Verification items for the finished model (mm, model axes). A direction names the side the tool comes from. Give positions to 0.01 mm unless a question says otherwise; leave off trailing zeros. Loops run counter-clockwise (first coordinate to the right, second up) from the corner with the lowest first, then second, coordinate; pieces in that order, holes last. Notation, with made-up numbers: M 16,-10.5 L 57,-10.5 A24 ccw 57,26.5 Z; hole C 39.25,-13 d6. An arc over 180 degrees is marked long. Use CSV: the item, a comma, the result in double quotes.
from build123d import *

# Parameters (mm, degrees)
SKETCH1_W         = 67.6
SKETCH1_H         = 30
SUBSTRATE_DEPTH   = 1.4
SKETCH2_R         = 1
SKETCH2_R_2       = 0.75
SKETCH2_R_3       = 1.75
CUTOUTS_DEPTH     = 2
SKETCH3_W         = 12.009016129
SKETCH3_H         = 11.886366808
SKETCH3_W_2       = 10.970861006
SKETCH3_H_2       = 9.979144757
CHIPS_DEPTH       = 0.3
SKETCH4_W         = 3.027468224
SKETCH4_H         = 1.391658781
SKETCH4_H_2       = 1.39165878
SKETCH4_W_2       = 1.760997679
SKETCH4_H_3       = 0.651327909
SKETCH4_W_3       = 1.447395353
SKETCH4_H_4       = 3.063653498
SKETCH4_W_4       = 1.857490704
SKETCH4_H_5       = 4.173323269
SKETCH4_H_6       = 4.331448702
SKETCH4_W_5       = 1.380452242
SKETCH4_H_7       = 0.625805016
CAPACITORS_DEPTH  = 0.5
SKETCH5_W         = 1.436881646
SKETCH5_H         = 0.57938776
SKETCH5_H_2       = 0.602563271
SKETCH5_H_3       = 0.695265312
SKETCH5_H_4       = 0.672089802
SKETCH5_W_2       = 1.465504975
SKETCH5_H_5       = 0.595361396
SKETCH5_W_3       = 1.305099019
SKETCH5_H_6       = 0.770620802
RESISTORS_DEPTH   = 0.3
SKETCH6_W         = 1.05591146
SKETCH6_H         = 1.163292287
SKETCH6_W_2       = 0.966427438
SKETCH6_W_3       = 1.020117852
SKETCH6_W_4       = 1.020117851
L_COMPONENT_DEPTH = 0.3


with BuildPart() as part:
    # Sketch1 → Substrate (new body)
    with BuildSketch(Plane.XY):
        Rectangle(SKETCH1_W, SKETCH1_H)
    extrude(amount=SUBSTRATE_DEPTH)

    # Sketch2 → Cutouts (cut)
    with BuildSketch(Plane.XY.offset(1.4)):
        with Locations((-30.709168608, 11.804578588)):
            Circle(SKETCH2_R)
        with Locations((30.516911038, 11.804578588)):
            Circle(SKETCH2_R)
        with Locations((31.687531572, -8.991184565)):
            Circle(SKETCH2_R_2)
        with Locations((-31.899083746, -8.991184565)):
            Circle(SKETCH2_R_2)
        with Locations((-33.643638543, 4.936384587)):
            Circle(SKETCH2_R_3)
        with Locations((33.376123728, 4.936384587)):
            Circle(SKETCH2_R_3)
        with BuildLine():
            Line((-18.1, -15), (-18.1, -11.517203937))
            ThreePointArc((-18.1, -11.517203937), (-17.7, -11.117203937), (-17.3, -11.517203937))
            Line((-17.3, -11.517203937), (-17.3, -15))
            Line((-17.3, -15), (-18.1, -15))
        make_face()
        with BuildLine():
            Line((33.057190194, -0.69758335), (34.638090789, -0.69758335))
            Line((34.638090789, -0.69758335), (34.710836401, -6.89758335))
            Line((34.710836401, -6.89758335), (33.057190194, -6.89758335))
            ThreePointArc((33.057190194, -6.89758335), (32.207190194, -6.04758335), (33.057190194, -5.19758335))
            Line((33.057190194, -5.19758335), (33.057190194, -2.39758335))
            ThreePointArc((33.057190194, -2.39758335), (32.207190194, -1.54758335), (33.057190194, -0.69758335))
        make_face()
        with BuildLine():
            Line((-33.341181022, -5.19758335), (-33.341181022, -2.39758335))
            ThreePointArc((-33.341181022, -2.39758335), (-32.491181022, -1.54758335), (-33.341181022, -0.69758335))
            Line((-33.341181022, -0.69758335), (-34.347477131, -0.69758335))
            Line((-34.347477131, -0.69758335), (-34.347477131, -6.89758335))
            Line((-34.347477131, -6.89758335), (-33.341181022, -6.89758335))
            ThreePointArc((-33.341181022, -6.89758335), (-32.491181022, -6.04758335), (-33.341181022, -5.19758335))
        make_face()
    extrude(amount=-CUTOUTS_DEPTH, mode=Mode.SUBTRACT)

    # Sketch3 → Chips (add)
    with BuildSketch(Plane.XY.offset(1.4)):
        with Locations((8.608474284, 3.159777946)):
            Rectangle(SKETCH3_W, SKETCH3_H)
        with Locations((-15.835757789, 3.059690457)):
            Rectangle(SKETCH3_W_2, SKETCH3_H_2)
    extrude(amount=CHIPS_DEPTH)

    # Sketch4 → Capacitors (add)
    with BuildSketch(Plane.XY.offset(1.4)):
        with Locations((10.666269416, 12.728744546)):
            Rectangle(SKETCH4_W, SKETCH4_H)
        with Locations((10.666269416, 10.677878974)):
            Rectangle(SKETCH4_W, SKETCH4_H_2)
        with Locations((18.085628066, 9.196485107)):
            Rectangle(SKETCH4_W_2, SKETCH4_H_3)
        with Locations((26.082487394, -3.540594003)):
            Rectangle(SKETCH4_W_3, SKETCH4_H_4)
        with Locations((28.579244378, -2.985759118)):
            Rectangle(SKETCH4_W_4, SKETCH4_H_5)
        with Locations((28.579244378, -8.450852566)):
            Rectangle(SKETCH4_W_4, SKETCH4_H_6)
        with Locations((26.082487394, -8.450852566)):
            Rectangle(SKETCH4_W_3, SKETCH4_H_6)
        with Locations((18.124891861, 4.272795947)):
            Rectangle(SKETCH4_W_5, SKETCH4_H_7)
    extrude(amount=CAPACITORS_DEPTH)

    # Sketch5 → Resistors (add)
    with BuildSketch(Plane.XY.offset(1.4)):
        with Locations((18.11021309, 8.134894019)):
            Rectangle(SKETCH5_W, SKETCH5_H)
        with Locations((18.11021309, 7.034057275)):
            Rectangle(SKETCH5_W, SKETCH5_H_2)
        with Locations((18.11021309, 5.921632774)):
            Rectangle(SKETCH5_W, SKETCH5_H_3)
        with Locations((18.11021309, 3.128983768)):
            Rectangle(SKETCH5_W, SKETCH5_H_4)
        with Locations((17.571973081, -3.598556709)):
            Rectangle(SKETCH5_W_2, SKETCH5_H_5)
        with Locations((0.65254951, 3.128983768)):
            Rectangle(SKETCH5_W_3, SKETCH5_H_4)
        with Locations((17.571973081, -2.438862849)):
            Rectangle(SKETCH5_W_2, SKETCH5_H_6)
    extrude(amount=RESISTORS_DEPTH)

    # Sketch6 → L Component (add)
    with BuildSketch(Plane.XY.offset(1.4)):
        with Locations((5.21332261, -9.903818455)):
            Rectangle(SKETCH6_W, SKETCH6_H)
        with Locations((6.994054649, -9.903818455)):
            Rectangle(SKETCH6_W_2, SKETCH6_H)
        with Locations((8.774786688, -9.903818455)):
            Rectangle(SKETCH6_W_3, SKETCH6_H)
        with Locations((10.600260739, -9.903818455)):
            Rectangle(SKETCH6_W_4, SKETCH6_H)
    extrude(amount=L_COMPONENT_DEPTH)


solid = part.part
(1) Section check A-A on y = 0.5. Record the cut outline in (x, z).
Calculated:
outline,"M -33.8,0 L 33.8,0 L 33.8,1.4 L 14.61,1.4 L 14.61,1.7 L 2.6,1.7 L 2.6,1.4 L -10.35,1.4 L -10.35,1.7 L -21.32,1.7 L -21.32,1.4 L -33.8,1.4 Z"
(2) Section check B-B on x = -2. Record the cut outline in (y, z), plus the area to 3 significant figures.
Calculated:
outline,"M -15,0 L 15,0 L 15,1.4 L -15,1.4 Z"
area,"42.0 mm²"
(3) Tool access check on faces 1 (the flat face through (9, 3, 1.7)), 2 (the flat face through (-33.341, -4, 1)), 3 (the flat face through (-17.3, -13, 1)), 4 (the cylindrical face through (32.207, -1.566, 0.71)). Record the directions out of +Z, -Z, +X, -X, +Y, -Y that give a thin tool (end or side, any length) a straight path to the whole face; none if there is none.
Calculated:
face 1,"+Z, -X, -Y"
face 2,"+Z, -Z, -X"
face 3,"+Z, -Z, -Y"
face 4,"+Z, -Z, +X"
(4) Scan lines: L1, parallel to X at y = -9, z = 0.9; L2, parallel to X at y = 1.25, z = 1.65; L3, parallel to X at y = -8.75, z = 1.2. Record each from-to range of solid material in increasing order. Write a range as from..to.
Calculated:
L1,"x = -33.8..-32.65, -31.15..30.94, 32.44..33.8"
L2,"x = -21.32..-10.35, 2.6..14.61"
L3,"x = -33.8..-32.61, -31.19..30.98, 32.4..33.8"
(5) Depth check by flat-ended pin: pin 1 Ø1.2 at (x, y) = (-30.71, 11.8) entering from +Z; pin 2 Ø0.6 at (x, y) = (18, 6) entering from +Z. Enter the tip coordinate at first touch or a pass-through.
Calculated:
pin 1,"passes through"
pin 2,"stops at z = 1.7"
(6) Mould release check, pull along Y, two halves, no side actions. Record for faces 5 (the cylindrical face through (-31.894, 4.896, 0.71)), 6 (the flat face through (-26, -15, 1)), 7 (the flat face through (-16, 3, 1.7)): released by +Y, released by -Y, zero draft, split by the parting line, or undercut.
Calculated:
face 5,"undercut"
face 6,"released by -Y"
face 7,"zero draft"
